Autodesk Inventor part; units mm, degrees
ref_plane "YZ Plane" through (0, 0, 0) normal (1, 0, 0) x (0, 1, 0)
ref_plane "XZ Plane" through (0, 0, 0) normal (0, 1, 0) x (-1, 0, 0)
ref_plane "XY Plane" through (0, 0, 0) normal (0, 0, 1) x (1, 0, 0)
sketch "Sketch1" plane through (0, 0, 0) normal (0, 1, 0) x (-1, 0, 0)
  line L0 (22.7522, 7.5) -> (-27.7522, 7.5)
  line L1 (-27.7522, 7.5) -> (-27.7522, 6)
  line L2 (-27.7522, 6) -> (17.7478, 6)
  line L3 (17.7478, 6) -> (20.7522, 1)
  line L4 (20.7522, 1) -> (27.7522, 1)
  line L5 (27.7522, 1) -> (27.7522, 1.75)
  line L6 (27.7522, 1.75) -> (22.7522, 1.75)
  line L7 (22.7522, 1.75) -> (22.7522, 7.5)
  line L8 (27.7522, 0) -> (-27.7522, 0)
  point P0 (0, 0)
  point P1 (0, 0)
  dimension "d0" = 2
  dimension "d1" = 3.5
  dimension "d2" = 5
  dimension "d3" = 59
  dimension "d5" = 1.5
  dimension "d6" = 2
  dimension "d13" = 12
  dimension "d14" = 45.5
revolve "Revolution1" add sketch "Sketch1" angle 360 about axis through (-27.7522, 0, 0) along (1, 0, 0)
fillet "Fillet1" radius 1 1 edges at (-22.7522, 0, -1.75)
fillet "Fillet1" radius 0.25 2 edges at (-27.7522, 0, -1.75) (-27.7522, 0, -1)
thread "Thread1"
properties part number "PayloadGermination_Syringe" material "Polycarbonate, Clear"
Verification items for the finished model (mm, model axes). A direction names the side the tool comes from. Give positions to 0.01 mm unless a question says otherwise; leave off trailing zeros. Loops run counter-clockwise (first coordinate to the right, second up) from the corner with the lowest first, then second, coordinate; pieces in that order, holes last. Notation, with made-up numbers: (-39, 87.5) - (-7, 87.5) arc R15 ccw to (-7, 100.5) - close; hole circle Ø10 at (76, -32). An arc over 180 degrees is marked (long way). Write each question's results on one line, items separated by ' | '.
1) Sectioned sample at C-C on x = -2. Record the boundary of the cut face in (y, z).
Solution:
outline: circle Ø15 at (0, 0); hole circle Ø12 at (0, 0)
2) Material ranges on L1, parallel to Z at x = 14, y = 0; L2, parallel to Y at x = -23.75, z = 0; L3, parallel to Y at x = -22.25, z = 0, recorded low to high. Write a range as from..to.
Solution:
L1: -7.5..-6, 6..7.5 | L2: -1.75..-1, 1..1.75 | L3: -7.5..-1, 1..7.5
3) Mould release check, pull along Y, two halves, no side actions. Record for faces 4 (the flat face through (-22.752, 3, 0)), 5 (the cylindrical face through (-24, -1, 0)), 6 (the cylindrical face through (2.854, -0.33, -7.493)): pulls with the +Y half, pulls with the -Y half, needs draft (parallel to the pull), parting line crosses it, or undercut.
Solution:
face 4: needs draft | face 5: undercut | face 6: parting line crosses it
4) Depth check by flat-ended pin: P1, Ø1, axis at x = 6.5, z = -5, coming from the +Y side; P2, Ø4, axis at y = 2, z = -5.5, coming from the -X side; P3, Ø2.5, axis at y = 0, z = 0, coming from the +X side. Enter the tip coordinate at first touch or a pass-through.
Solution:
P1: y = 6 | P2: x = -22.75 | P3: x = -20.6
5) Tool access check on faces 1 (the cylindrical face through (5, 0, -6)), 2 (the flat face through (27.752, -6, 2)), 3 (the cylindrical face through (-25.601, 0.67, 1.617)). Record the directions out of +Z, -Z, +X, -X, +Y, -Y that give a thin tool (end or side, any length) a straight path to the whole face; none if there is none.
Solution:
face 1: +X | face 2: +Z, -Z, +X, +Y, -Y | face 3: -X
6) Sectioned sample at A-A on z = 0. Record the boundary of the cut face in (x, y), plus the area to 3 significant figures.
Solution:
outline: (-27.75, -1.5) arc R0.25 ccw to (-27.5, -1.75) - (-23.75, -1.75) arc R1 cw to (-22.75, -2.75) - (-22.75, -7.5) - (27.75, -7.5) - (27.75, -6) - (-17.75, -6) - (-20.75, -1) - (-27.5, -1) arc R0.25 ccw to (-27.75, -1.25) - close; (-27.75, 1.25) arc R0.25 ccw to (-27.5, 1) - (-20.75, 1) - (-17.75, 6) - (27.75, 6) - (27.75, 7.5) - (-22.75, 7.5) - (-22.75, 2.75) arc R1 cw to (-23.75, 1.75) - (-27.5, 1.75) arc R0.25 ccw to (-27.75, 1.5) - close | area: 194 mm2
